Autodesk Inventor part; units mm, degrees
ref_plane "YZ Plane" through (0, 0, 0) normal (1, 0, 0) x (0, 1, 0)
ref_plane "XZ Plane" through (0, 0, 0) normal (0, 1, 0) x (-1, 0, 0)
ref_plane "XY Plane" through (0, 0, 0) normal (0, 0, 1) x (1, 0, 0)
sketch "Sketch1" plane through (0, 0, 0) normal (0, 1, 0) x (-1, 0, 0)
  line L0 (-20, 0) -> (0, 0)
  line L1 (0, 0) -> (0, -29.5)
  line L2 (0, -29.5) -> (-20, -29.5)
  line L3 (-20, -29.5) -> (-20, 0)
  dimension "d1" = 20
  dimension "d2" = 29.5
sketch "Sketch2" plane through (0, 0, 0) normal (0, 0, 1) x (1, 0, 0)
  point P0 (0, 0)
extrude "Extrusion1" add sketch "Sketch1" along normal blind 2
sketch "Sketch3" plane through (0, 0, 0) normal (0, 0, 1) x (1, 0, 0)
  line L0 (20, 0) -> (0, 0)
  line L1 (0, 0) -> (20, 0)
  line L2 (20, 0) -> (20, 10)
  line L3 (20, 10) -> (0, 10)
  line L4 (0, 10) -> (0, 0)
  dimension "d11" = 10
extrude "Extrusion2" add sketch "Sketch3" along normal blind 2
sketch "Sketch4" plane through (0, 0, 2) normal (0, 0, 1) x (1, 0, 0)
  circle A0 centre (5.25, 7.5) radius 2.5
  circle A1 centre (14.75, 7.5) radius 2.5
  line L0 (20, 10) -> (0, 10)
  line L1 (0, 10) -> (0, 0)
  dimension "d18" = 5
  dimension "d19" = 5
  dimension "d20" = 2.5
  dimension "d21" = 2.5
  dimension "d22" = 9.5
  dimension "d23" = 5.25
extrude "Extrusion3" cut sketch "Sketch4" against normal blind 2 contours A1
sketch "Sketch5" plane through (0, 0, 2) normal (0, 0, 1) x (1, 0, 0)
  circle A0 centre (5.25, 7.5) radius 2.5
  line L0 (14.75, 10) -> (0, 10)
  circle A1 centre (14.75, 7.5) radius 2.5
  point P0 (0, 0)
  dimension "d26" = 5
  dimension "d27" = 2.5
  dimension "d28" = 9.5
extrude "Extrusion4" cut sketch "Sketch5" against normal blind 2 contours A0
sketch "Sketch7" plane through (20, 0, -29.5) normal (0, 0, -1) x (-1, 0, 0)
  line L0 (20, 0) -> (0, 0)
  line L1 (0, 0) -> (20, 0)
  line L2 (20, 0) -> (20, 20)
  line L3 (20, 20) -> (0, 20)
  line L4 (0, 20) -> (0, 0)
  dimension "d34" = 20
extrude "Extrusion6" add sketch "Sketch7" along normal blind 2
properties part number "Servo Holder Bottom"
Could you check a few things on this model? Use its own coordinates, in mm. A direction names the side the tool comes from. Give positions to 0.01 mm unless a question says otherwise; leave off trailing zeros. Loops run counter-clockwise (first coordinate to the right, second up) from the corner with the lowest first, then second, coordinate; pieces in that order, holes last. Notation, with made-up numbers: (-26.5, -36.5) -> (22.5, -36.5) arc R9 cw to (22.5, -31.5) -> close; hole circle Ø1 at (39.5, 51). An arc over 180 degrees is marked (long way). Return JSON: item names as keys, results as strings.
Item 1: I'm going to push flat-ended pins straight in: pin 1 (12 mm diameter, centred on x = 11.5, z = -14, fed in from +Y); pin 2 (12 mm diameter, centred on y = 15.5, z = -9, fed in from -X); pin 3 (0.6 mm diameter, centred on x = 3, z = 1, fed in from +Y). Where does each tip first touch, or does it pass through?
Geometry results:
{"pin 1": "stops at y = 2", "pin 2": "passes through", "pin 3": "stops at y = 10"}
Item 2: I need wall thicknesses on L1, parallel to X at y = 7.5, z = 0.45; L2, parallel to Z at x = 7, y = 5; L3, parallel to Y at x = 15.5, z = -7.5. Which ranges of each line are inside material? Lowest first, please. Write a range as from..to.
Geometry results:
{"L1": "x = 0..2.75, 7.75..12.25, 17.25..20", "L2": "z = -31.5..-29.5, 0..2", "L3": "y = 0..2"}
Item 3: If we section it at A-A on y = 2.75: List the corners of the cut face in (x, z) for me.
Geometry results:
{"outline": "(0, -31.5) -> (20, -31.5) -> (20, -29.5) -> (0, -29.5) -> close; (0, 0) -> (20, 0) -> (20, 2) -> (0, 2) -> close"}
Item 4: If we section it at D-D on x = 16.5: List the corners of the cut face in (y, z) for me, plus the area to 3 significant figures.
Geometry results:
{"outline": "(0, -31.5) -> (20, -31.5) -> (20, -29.5) -> (2, -29.5) -> (2, 0) -> (5.71, 0) -> (5.71, 2) -> (0, 2) -> close; (9.29, 0) -> (10, 0) -> (10, 2) -> (9.29, 2) -> close", "area": "112 mm²"}
Item 5: If we section it at B-B on y = 6: List the corners of the cut face in (x, z) for me, plus the area to 3 significant figures.
Geometry results:
{"outline": "(0, -31.5) -> (20, -31.5) -> (20, -29.5) -> (0, -29.5) -> close; (0, 0) -> (3.25, 0) -> (3.25, 2) -> (0, 2) -> close; (7.25, 0) -> (12.75, 0) -> (12.75, 2) -> (7.25, 2) -> close; (16.75, 0) -> (20, 0) -> (20, 2) -> (16.75, 2) -> close", "area": "64.0 mm²"}
Item 6: If we section it at C-C on x = 9: List the corners of the cut face in (y, z) for me.
Geometry results:
{"outline": "(0, -31.5) -> (20, -31.5) -> (20, -29.5) -> (2, -29.5) -> (2, 0) -> (10, 0) -> (10, 2) -> (0, 2) -> close"}
Item 7: Which directions (+Z, -Z, +X, -X, +Y, -Y) give clear straight access to the entire face, cutting with the end or side of a thin tool? Please do faces 1 (the flat face through (10, 10, 1)), 2 (the flat face through (20, 1, -17)), 3 (the flat face through (10, 2, -15)).
Geometry results:
{"face 1": "+Z, +X, -X, +Y", "face 2": "+Z, -Z, +X, +Y, -Y", "face 3": "+X, -X, +Y"}
Item 8: We'd pull the mould along Z, two halves only. Please class faces 4 (the flat face through (17, 10, 1)), 5 (the flat face through (10, 5, 0)), 6 (the flat face through (10, 4, 2)), 7 (the flat face through (10, 11, -29.5)): +Z half, -Z half, draft (parallel to the pull), parting line (faces both ways), or undercut.
Geometry results:
{"face 4": "draft", "face 5": "undercut", "face 6": "+Z half", "face 7": "undercut"}
